For this review, use the dimensioned drawing (mm, ordinates from the lowest corner) and the shaded views. A direction names the side the tool comes from. Round coordinates to 2 decimals unless told otherwise and drop trailing zeros. Order: outer loops, then holes, each group sorted by start corner. A loop starts at its lowest first (then second) coordinate and runs counter-clockwise, first axis right, second up. Notation, with made-up numbers: (69.25, -1.75) - (77.25, -1.75) arc R37 cw to (77.25, 37.25) - close; hole circle Ø2 at (-27.5, 63.5). An arc over 180 degrees is marked (long way). Write each question's results on one line, items separated by ' | '. Start each with the question number.
(1) Take a section at C-C, the plane x = 4. Give the boundary of the cut face in (y, z), plus the area to 3 significant figures.
(2) Insertion check: pin 1 Ø8 at (y, z) = (15, 14) entering from -X; pin 2 Ø6 at (x, y) = (18.5, 8) entering from -Z; pin 3 Ø5 at (x, z) = (2, 31) entering from -Y; pin 4 Ø5 at (x, z) = (36, 66.5) entering from +Y. Each pin has a flat end and moves straight along its axis. Give the tip position at first contact, or say it passes through.
(3) Take a section at B-B, the plane y = 20.5. Give the boundary of the cut face in (x, z), plus the area to 3 significant figures.
(4) Take a section at D-D, the plane z = 16. Give the boundary of the cut face in (x, y), plus the area to 3 significant figures.
(5) For L1, parallel to Y at x = 4, z = 43; L2, parallel to X at y = 13.5, z = 53; L3, parallel to Z at x = 23.5, y = 9.5, list the stretches that pass through material, from the lowest coordinate up. Write a range as from..to.
(6) Take a section at A-A, the plane z = 65.5. Give the boundary of the cut face in (x, y).
(7) For the marked faces 1, 2 and 3, list the 3-axis set-ups (+Z, -Z, +X, -X, +Y, -Y) from which the entire face can be reached by the end or side of a thin tool; tool diameter is ignored.
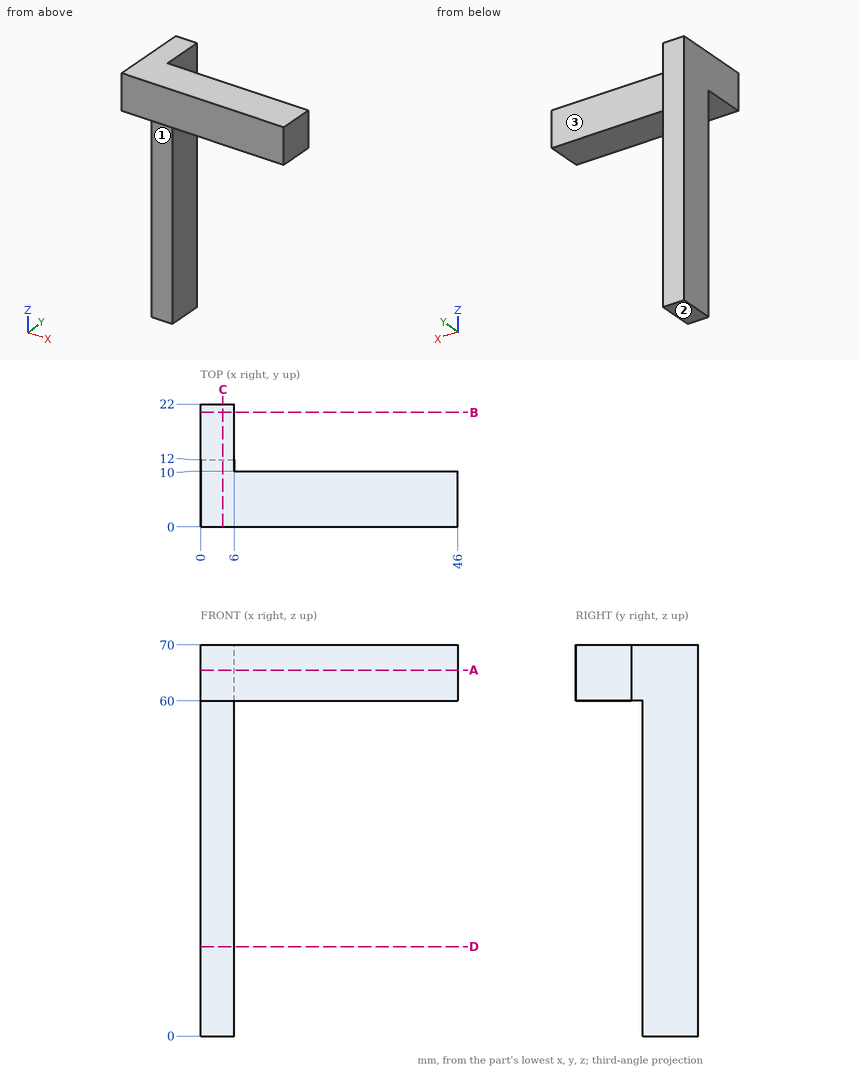
Results below:
1) outline: (0, 60) - (12, 60) - (12, 0) - (22, 0) - (22, 70) - (0, 70) - close | area: 820 mm^2
2) pin 1: stops at x = 0 | pin 2: stops at z = 60 | pin 3: stops at y = 12 | pin 4: stops at y = 10
3) outline: (0, 0) - (6, 0) - (6, 70) - (0, 70) - close | area: 420 mm^2
4) outline: (0, 12) - (6, 12) - (6, 22) - (0, 22) - close | area: 60.0 mm^2
5) L1: y = 12..22 | L2: x = 0..6 | L3: z = 60..70
6) outline: (0, 0) - (46, 0) - (46, 10) - (6, 10) - (6, 22) - (0, 22) - close
7) face 1: -Z, +X, -X, -Y | face 2: -Z, +X, -X, +Y, -Y | face 3: +Z, -Z, +X, +Y
